from build123d import *

# Parameters (mm, degrees)
FILLET1_R           = 5
BOSS_EXTRUDE1_REACH = 306.713
CIRPATTERN1_COUNT   = 3


with BuildPart() as part:
    # Sketch1 → Revolve1 (revolve)
    with BuildSketch(Plane.XY, mode=Mode.PRIVATE) as revolve1_sk:
        Polygon((-70, 0), (-85, 0), (-85, 15), (-30, 245), (-30, 260), (-15, 260), (-15, 245), (-70, 15), align=None)
    revolve(revolve1_sk.sketch.rotate(Axis((0, 0, 0), (0, 1, 0)), 270), axis=Axis((0, 0, 0), (0, 1, 0)))

    # Fillet1
    fillet1_edges = [part.edges().sort_by_distance(p)[0] for p in [
        (0, 0, 70),
        (0, 0, 85),
    ]]
    fillet(fillet1_edges, radius=FILLET1_R)



with BuildPart() as body_2:
    # Sketch3 → Revolve2 (revolve)
    with BuildSketch(Plane.XY, mode=Mode.PRIVATE) as revolve2_sk:
        with BuildLine():
            Line((0, 30), (0, 280))
            Line((0, 280), (-20, 50))
            ThreePointArc((-20, 50), (-14.142135624, 35.857864376), (0, 30))
        make_face()
    revolve(revolve2_sk.sketch.rotate(Axis((0, 50, 0), (0, 1, 0)), 90), axis=Axis((0, 50, 0), (0, 1, 0)))


with BuildPart() as part_1:
    add(part.part)

    add(body_2.part)  # Boss-Extrude1 merges body 2
    # Boss-Extrude1: up to this cone (the profile starts inside it)
    boss_extrude1_end = Plane(origin=(0, 102, 0), z_dir=(0, -1, 0)).offset(-205.727271727) * Cone(1e-06, 134.423808129, 562.135923901, align=(Align.CENTER, Align.CENTER, Align.MIN), mode=Mode.PRIVATE)
    # Sketch5 → Boss-Extrude1 (add, up to the surface)
    with BuildSketch(Plane(origin=(0, 0, 0), x_dir=(0, 0, -1), z_dir=(1, 0, 0)), mode=Mode.PRIVATE) as boss_extrude1_sk1:
        with BuildLine():
            Line((-1, 62), (1, 62))
            ThreePointArc((1, 62), (4.535533906, 63.464466094), (6, 67))
            Line((6, 67), (6, 137))
            ThreePointArc((6, 137), (4.535533906, 140.535533906), (1, 142))
            Line((1, 142), (-1, 142))
            ThreePointArc((-1, 142), (-4.535533906, 140.535533906), (-6, 137))
            Line((-6, 137), (-6, 67))
            ThreePointArc((-6, 67), (-4.535533906, 63.464466094), (-1, 62))
        make_face()
    boss_extrude1_tool1 = extrude(boss_extrude1_sk1.sketch, amount=BOSS_EXTRUDE1_REACH, mode=Mode.PRIVATE) & boss_extrude1_end
    boss_extrude1 = boss_extrude1_tool1.solids().sort_by_distance((0, 102, 0))[0]
    add(boss_extrude1)

    # CirPattern1: Boss-Extrude1 ×3 about axis
    cirpattern1_axis = Axis((0, 0, 0), (0, 1, 0))
    for i in range(1, CIRPATTERN1_COUNT):
        add(boss_extrude1.rotate(cirpattern1_axis, i * 360 / CIRPATTERN1_COUNT))


solid = part_1.part
Can you work these out from the model? Positions are in its coordinate system, mm. A direction names the side the tool comes from. Coordinates: 2 decimals unless noted, no trailing zeros. Write each loop counter-clockwise with the first axis right and the second up, starting at its lowest first coordinate (ties: lowest second). Pieces come first, ordered by that corner, then holes. Notation, with made-up numbers: (42, 45) - (74, 45) arc R15 cw to (74, 68) - close; hole circle Ø11 at (-6.5, -24). An arc over 180 degrees is marked (long way). Return JSON: item names as keys, results as strings. Group by question number.
Item 1: We'd pull the mould along Z, two halves only. Please class faces 3 (the face through (-1.32, 252.6, 29.97)), 4 (the face through (34, 102, 6)), 5 (the face through (26.095, 128.39, 34.032)): pulls with the +Z half, pulls with the -Z half, needs draft (parallel to the pull), parting line crosses it, or undercut.
Item 2: If we section it at C-C (y = 181.5): Write out the boundary of the cut face in (x, z).
Item 3: If we section it at B-B (y = 104): Write out the boundary of the cut face in (x, z).
Item 4: I'm going to push flat-ended pins straight in: pin 1 Ø1.6 at (x, z) = (37, 0.5) entering from -Y; pin 2 Ø14 at (x, y) = (41.5, 117.5) entering from +Z; pin 3 Ø6 at (x, y) = (-3, 165.5) entering from -Z. Where does each tip first touch, or does it pass through?
Item 5: Which directions (+Z, -Z, +X, -X, +Y, -Y) give clear straight access to the entire face, cutting with the end or side of a thin tool? Please do faces 1 (the face through (-11.68, 101.51, 32.23)), 2 (the face through (51.721, 10.07, 67.453)).
Item 6: If we section it at A-A (y = 39): Write out the boundary of the cut face in (x, z), then the cut area to 3 significant figures.
Item 7: Please list where these lines run through material, in increasing order: probe 1 along Z at (x, y) = (40.5, 115); probe 2 along X at (y, z) = (252, 0); probe 3 along Z at (x, y) = (1, 121).
Return value:
{
 "1": {"face 3": "parting line crosses it", "face 4": "undercut", "face 5": "undercut"},
 "2": {"outline": "circle Ø90.37 at (0, 0); circle Ø17.13 at (0, 0); hole circle Ø60.37 at (0, 0)"},
 "3": {"outline": "circle Ø127.43 at (0, 0); hole (-29.37, -38.87) - (-12.24, -9.19) arc R15.3 cw to (-12.24, 9.19) - (-29.37, 38.87) arc R48.72 ccw to start; hole (-18.98, -44.87) arc R48.72 ccw to (48.35, -6) - (14.08, -6) arc R15.3 cw to (-1.84, -15.19) - close; hole (-18.98, 44.87) - (-1.84, 15.19) arc R15.3 cw to (14.08, 6) - (48.35, 6) arc R48.72 ccw to start"},
 "4": {"pin 1": "stops at y = 62", "pin 2": "stops at z = 50.1", "pin 3": "stops at z = -49.66"},
 "5": {"face 1": "none", "face 2": "+Y, -Y"},
 "6": {"outline": "circle Ø158.52 at (0, 0); circle Ø33.41 at (0, 0); hole circle Ø128.52 at (0, 0)", "area": "7,640 mm^2"},
 "7": {"probe 1": "z = -45.73 to -21.99, -6 to 6, 21.99 to 45.73", "probe 2": "x = -30 to -15, -2.43 to 2.43, 15 to 30", "probe 3": "z = -59.64 to -44.64, -13.79 to 13.79, 44.64 to 59.64"}
}
